Read the model definition and answer for the solid it produces. Units are mm, in the model's axes. A direction names the side the tool comes from. Coordinates: 2 decimals unless noted, no trailing zeros. Write each loop counter-clockwise with the first axis right and the second up, starting at its lowest first coordinate (ties: lowest second). Pieces come first, ordered by that corner, then holes. Notation, with made-up numbers: (75, -24.5) -> (116, -24.5) arc R18 cw to (116, -8.5) -> close; hole circle Ø2 at (68, 23.5). An arc over 180 degrees is marked (long way). Answer as a JSON object with one key per item and string values. Group by question number.
(1) Flat-ended cylindrical pins translate along their axes: P1, Ø1.5, axis at y = 16, z = 7.5, coming from the +X side; P2, Ø12, axis at x = 24, z = 15, coming from the +Y side; P3, Ø1.5, axis at y = -33.5, z = 18, coming from the +X side. Find the tip coordinate at first contact, or state that the pin passes through.
(2) Straight lines are drawn through the part: L1, parallel to Z at x = -14, y = 18.5; L2, parallel to X at y = 4, z = 14.5; L3, parallel to X at y = -10.5, z = 27.5. For each, find the intervals that lie inside material, in ascending order.
(3) For a pull along X with two mould halves and no side action, classify faces 4 (the face through (15.369, -37.706, 20.902)), 5 (the face through (-3.076, 22.697, 9.07)), 6 (the face through (5.761, 9.926, 9.07)) as +X half, -X half, draft (parallel to the pull), parting line (faces both ways), or undercut.
(4) Which of the six approach directions +Z, -Z, +X, -X, +Y, -Y give full straight-line access (tool end or side, diameter ignored) to faces 1 (the face through (-5.761, -9.926, 9.07)), 2 (the face through (-22.697, -3.076, 9.07)), 3 (the face through (18.22, -13.87, 9.07))?
(5) Find section B-B (z = 25). Give the vertices of the cut face in (x, y), then the cut area to 3 significant figures.
(6) Find section A-A (z = 5.5). Count the separate pieces of the cut face and the enclosed holes in it, then the cut area to 3 significant figures.
from build123d import *

# Parameters (mm, degrees)
PAD003_DEPTH          = 15
PAD007_DEPTH          = 10
POLARPATTERN006_COUNT = 10
PAD008_DEPTH          = 10
POLARPATTERN007_COUNT = 16
FILLET001_R           = 1


with BuildPart() as part:
    # Sketch007 → Pad003 (new body)
    with BuildSketch(Plane.XY.offset(14)):
        Polygon((0, 44.072464), (-31.163938, 31.163938), (-44.072464, 0), (-31.163938, -31.163938), (0, -44.072464), (31.163938, -31.163938), (44.072464, 0), (31.163938, 31.163938), align=None)
    extrude(amount=PAD003_DEPTH)

    # Sketch015 (on Face9 of Pad003) → Pad007 (join)
    with BuildSketch(Plane(origin=(0, 0, 14), x_dir=(1, 0, 0), z_dir=(0, 0, -1))):
        Polygon((-10.494645, 8.088568), (-7.65128, 7.190822), (-7.65128, -1.233051), (-10.494645, -0.335305), align=None)
    pad007 = extrude(amount=PAD007_DEPTH)

    # PolarPattern006: Pad007 ×10 about axis
    polarpattern006_axis = Axis((0, 0, 14), (0, 0, -1))
    for i in range(1, POLARPATTERN006_COUNT):
        add(pad007.rotate(polarpattern006_axis, i * 360 / POLARPATTERN006_COUNT))

    # Sketch016 (on Face4 of PolarPattern006) → Pad008 (join)
    with BuildSketch(Plane(origin=(0, 0, 14), x_dir=(1, 0, 0), z_dir=(0, 0, -1))):
        Polygon((-24.069083, 2.956647), (-20.580814, -6.219331), (-17.772233, -5.975805), (-21.260501, 3.200173), align=None)
    pad008 = extrude(amount=PAD008_DEPTH)

    # PolarPattern007: Pad008 ×16 about axis
    polarpattern007_axis = Axis((0, 0, 14), (0, 0, -1))
    for i in range(1, POLARPATTERN007_COUNT):
        add(pad008.rotate(polarpattern007_axis, i * 360 / POLARPATTERN007_COUNT))

    # Fillet001
    fillet001_edges = [part.edges().sort_by_distance(p)[0] for p in [
        (-37.618201, 15.581969, 29),
        (-31.163938, 31.163938, 21.5),
        (-44.072464, 0, 21.5),
        (-37.618201, -15.581969, 29),
        (-31.163938, -31.163938, 21.5),
        (-15.581969, -37.618201, 29),
        (-15.581969, 37.618201, 29),
        (0, 44.072464, 21.5),
        (15.581969, 37.618201, 29),
        (0, -44.072464, 21.5),
        (15.581969, -37.618201, 29),
        (31.163938, -31.163938, 21.5),
        (37.618201, -15.581969, 29),
        (44.072464, 0, 21.5),
        (31.163938, 31.163938, 21.5),
        (37.618201, 15.581969, 29),
    ]]
    fillet(fillet001_edges, radius=FILLET001_R)


solid = part.part
Results below:
{
 "1": {"P1": "stops at x = 16.66", "P2": "stops at y = 36.62", "P3": "stops at x = 27.33"},
 "2": {"L1": "z = 14 to 29", "L2": "x = -42.42 to 42.42", "L3": "x = -39.72 to 39.72"},
 "3": {"face 4": "+X half", "face 5": "-X half", "face 6": "undercut"},
 "4": {"face 1": "-Z", "face 2": "-Z, -X, -Y", "face 3": "-Z, +X"},
 "5": {"outline": "(-43.91, -0.38) -> (-31.32, -30.78) arc R1 ccw to (-30.78, -31.32) -> (-0.38, -43.91) arc R1 ccw to (0.38, -43.91) -> (30.78, -31.32) arc R1 ccw to (31.32, -30.78) -> (43.91, -0.38) arc R1 ccw to (43.91, 0.38) -> (31.32, 30.78) arc R1 ccw to (30.78, 31.32) -> (0.38, 43.91) arc R1 ccw to (-0.38, 43.91) -> (-30.78, 31.32) arc R1 ccw to (-31.32, 30.78) -> (-43.91, 0.38) arc R1 ccw to start", "area": "5,490 mm2"},
 "6": {"separate pieces": "2", "enclosed holes": "2", "area": "645 mm2"}
}
